Could you check a few things on this drawing? It's one solid part, dimensions in mm from its lowest x, y, z. A direction names the side the tool comes from. Round coordinates to 2 decimals unless told otherwise and drop trailing zeros. Write each loop counter-clockwise with the first axis right and the second up, starting at its lowest first coordinate (ties: lowest second). Pieces come first, ordered by that corner, then holes. Notation, with made-up numbers: (13, -21) -> (52, -21) arc R21 cw to (52, 14) -> close; hole circle Ø5 at (-3.75, 67). An arc over 180 degrees is marked (long way). Put each result on its own line as item: value. Start each with the question number.
1) If I drill on line 1 along Z through (x, y) = (11, 21); line 2 along Y through (x, z) = (3.5, 26.5); line 3 along Z through (x, y) = (25.9, 21.7) (1 decimal), over which ranges is the centre line in solid material (lowest first)? Write a range as [from, to].
2) I want a section at A-A, the plane z = 18.5. List the corners of the cut face in (x, y) for me, then the cut area to 3 significant figures.
3) Will these pins go through, and if not, where does the flat tip stop? P1, Ø1.5, axis at y = 21.5, z = 26, coming from the +X side (1 decimal); P2, Ø4, axis at x = 11, z = 31.5, coming from the -Y side; P3, Ø1, axis at x = 10.5, z = 5.5, coming from the -Y side; P4, Ø6, axis at x = 6.5, y = 17, coming from the -Z side.
4) I want a section at B-B, the plane x = 18.5. List the corners of the cut face in (y, z) for me, then the cut area to 3 significant figures.
5) Which directions (+Z, -Z, +X, -X, +Y, -Y) give clear straight access to the entire face, cutting with the end or side of a thin tool? Please do the marked faces 1, 2, 3 and 4.
6) I want a section at D-D, the plane y = 23.5. List the corners of the cut face in (x, z) for me, then the cut area to 3 significant figures.
7) I want a section at C-C, the plane y = 58.5. List the corners of the cut face in (x, z) for me, then the cut area to 3 significant figures.
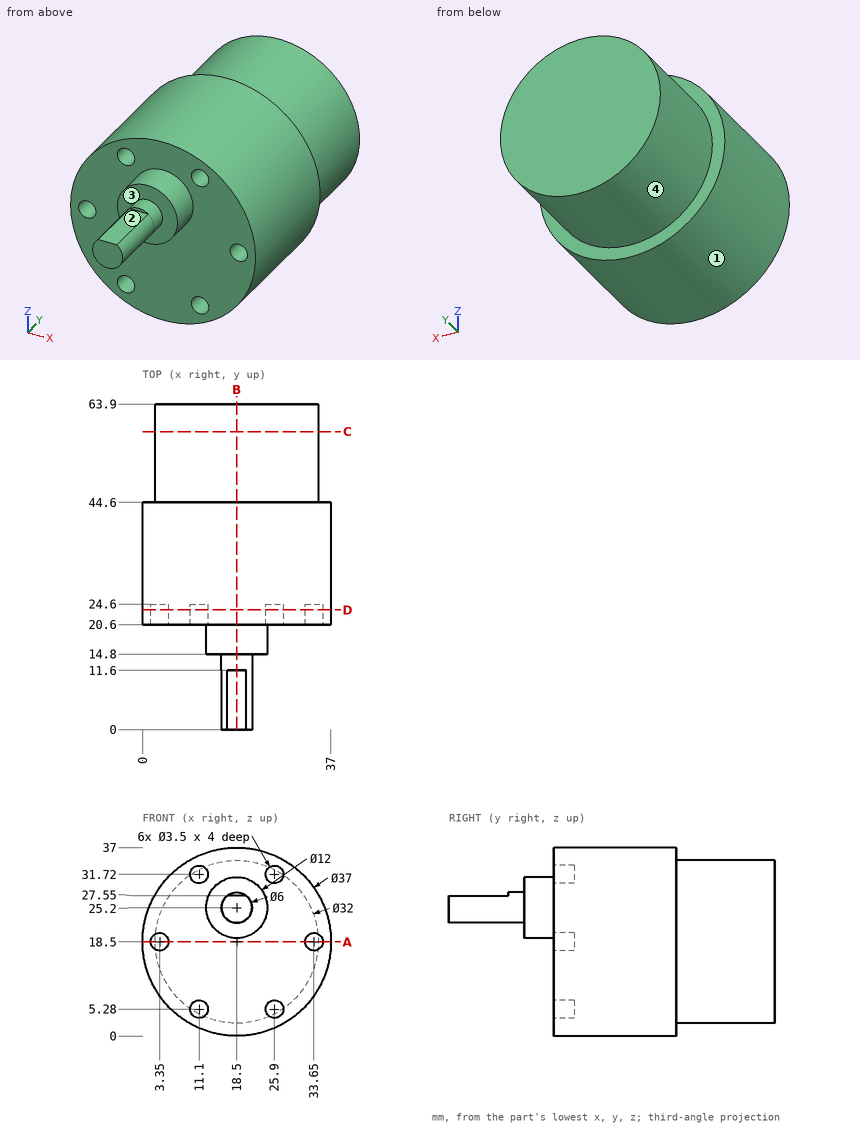
Findings:
1. line 1: z = [1.59, 3.53], [7.03, 29.97], [33.47, 35.41]
1. line 2: y = [20.6, 44.6]
1. line 3: z = [1.5, 3.5], [7, 30], [33.5, 35.5]
2. outline: (0, 20.6) -> (1.6, 20.6) -> (1.6, 24.6) -> (5.1, 24.6) -> (5.1, 20.6) -> (31.9, 20.6) -> (31.9, 24.6) -> (35.4, 24.6) -> (35.4, 20.6) -> (37, 20.6) -> (37, 44.6) -> (34.5, 44.6) -> (34.5, 63.9) -> (2.5, 63.9) -> (2.5, 44.6) -> (0, 44.6) -> close
2. area: 1,480 mm2
3. P1: stops at x = 35.7
3. P2: stops at y = 20.6
3. P3: stops at y = 24.6
3. P4: passes through
4. outline: (0, 22.2) -> (14.8, 22.2) -> (14.8, 19.2) -> (20.6, 19.2) -> (20.6, 0) -> (44.6, 0) -> (44.6, 2.5) -> (63.9, 2.5) -> (63.9, 34.5) -> (44.6, 34.5) -> (44.6, 37) -> (20.6, 37) -> (20.6, 31.2) -> (14.8, 31.2) -> (14.8, 28.2) -> (11.6, 28.2) -> (11.6, 27.55) -> (0, 27.55) -> close
4. area: 1,660 mm2
5. face 1: +Y, -Y
5. face 2: +Z, +X, -X, -Y
5. face 3: -Y
5. face 4: +Y
6. outline: circle Ø37 at (18.5, 18.5); hole circle Ø3.5 at (3.35, 18.5); hole circle Ø3.5 at (11.1, 5.28); hole circle Ø3.5 at (11.1, 31.72); hole circle Ø3.5 at (25.9, 5.28); hole circle Ø3.5 at (25.9, 31.72); hole circle Ø3.5 at (33.65, 18.5)
6. area: 1,020 mm2
7. outline: circle Ø32 at (18.5, 18.5)
7. area: 804 mm2
